Can you work these out from the model? Positions are in its coordinate system, mm. A direction names the side the tool comes from. Give positions to 0.01 mm unless a question says otherwise; leave off trailing zeros. Order: outer loops, then holes, each group sorted by start corner. A loop starts at its lowest first (then second) coordinate and runs counter-clockwise, first axis right, second up. Notation, with made-up numbers: (33.25, 56) - (69.25, 56) arc R5 cw to (69.25, 62) - close; hole circle Ø11 at (2.5, -31). An arc over 180 degrees is marked (long way). Use one line per item in the form item = value. Start each with the question number.
1) Suppose I cut it at A-A, the plane y = 17. Write out the boundary of the cut face in (x, z).
2) Which directions (+Z, -Z, +X, -X, +Y, -Y) give clear straight access to the entire face, cutting with the end or side of a thin tool? Please do faces 1 (the cylindrical face through (-0.22, 5.27, 1.97)), 2 (the flat face through (0, -26.786, 2)), 3 (the flat face through (-1, -14, 4)).
3) For pin 1 (2 mm diameter, centred on x = -14, z = 0.5, fed in from +Y); pin 2 (1.5 mm diameter, centred on x = -5, z = 3, fed in from -Y), each with a flat end and sliding along its axis, tell me the tip position at first contact or that it passes through.
4) Suppose I cut it at C-C, the plane z = 1.7. Write out the boundary of the cut face in (x, y), and give its area (3 significant figures).
5) Please list where these lines run through material, in increasing order: probe 1 along X at (y, z) = (20.5, 3.75); probe 2 along X at (y, z) = (0.5, 0.9); probe 3 along Y at (x, z) = (-24.5, 1.8).
6) Suppose I cut it at D-D, the plane y = 8. Write out the boundary of the cut face in (x, z).
7) We'd pull the mould along Y, two halves only. Please class faces 4 (the cylindrical face through (-35.992, -25.881, 1.972)), 5 (the flat face through (0, -13.786, 2)), 6 (the flat face through (-1, -14, 0)): released by +Y, released by -Y, zero draft, split by the parting line, or undercut.
8) Suppose I cut it at B-B, the plane x = 6.5. Write out the boundary of the cut face in (y, z), and give its area (3 significant figures).
```python
from build123d import *

# Parameters (mm, degrees)
SKETCH_1_R      = 5.2
EXTRUDE_1_DEPTH = 4


with BuildPart() as part:
    # 草图1 → 凸台-拉伸1 (new body)
    with BuildSketch(Plane.XY):
        with BuildLine():
            Line((-18.494622549, 4.742999843), (-23.409453688, -3.769737399))
            ThreePointArc((-23.409453688, -3.769737399), (-35.781809628, -26.257000157), (-10.121090849, -26.785856986))
            Line((-10.121090849, -26.785856986), (-0.291428571, -26.785856986))
            Line((-0.291428571, -26.785856986), (9.538233706, -26.785856986))
            ThreePointArc((9.538233706, -26.785856986), (35.198952485, -26.257000157), (22.826596545, -3.769737399))
            Line((22.826596545, -3.769737399), (17.911765406, 4.742999843))
            Line((17.911765406, 4.742999843), (12.996934268, 13.255737086))
            ThreePointArc((12.996934268, 13.255737086), (-0.291428571, 35.214143014), (-13.579791411, 13.255737086))
            Line((-13.579791411, 13.255737086), (-18.494622549, 4.742999843))
        make_face()
        with Locations((-0.291428571, 20.214143014)):
            Circle(SKETCH_1_R, mode=Mode.SUBTRACT)
        with Locations((22.208571429, -18.757000157)):
            Circle(SKETCH_1_R, mode=Mode.SUBTRACT)
        with Locations((-22.791428571, -18.757000157)):
            Circle(SKETCH_1_R, mode=Mode.SUBTRACT)
        with BuildLine():
            Line((9.268171867, -6.285856986), (4.038698447, 2.771856673))
            ThreePointArc((4.038698447, 2.771856673), (-0.291428571, 5.271856673), (-4.62155559, 2.771856673))
            Line((-4.62155559, 2.771856673), (-9.85102901, -6.285856986))
            ThreePointArc((-9.85102901, -6.285856986), (-9.85102901, -11.285856986), (-5.520901991, -13.785856986))
            Line((-5.520901991, -13.785856986), (4.938044848, -13.785856986))
            ThreePointArc((4.938044848, -13.785856986), (9.268171867, -11.285856986), (9.268171867, -6.285856986))
        make_face(mode=Mode.SUBTRACT)
    extrude(amount=EXTRUDE_1_DEPTH)


solid = part.part
```
Result sheet:
q1.outline = (-14.94, 0) - (-4.38, 0) - (-4.38, 4) - (-14.94, 4) - close; (3.8, 0) - (14.36, 0) - (14.36, 4) - (3.8, 4) - close
q2.face_1 = +Z, -Z
q2.face_2 = +Z, -Z, -Y
q2.face_3 = +Z, +X, -X, +Y, -Y
q3.pin_1 = 28.18
q3.pin_2 = -26.79
q4.outline = (-23.41, -3.77) arc R15 ccw (long way) to (-10.12, -26.79) - (9.54, -26.79) arc R15 ccw (long way) to (22.83, -3.77) - (13, 13.26) arc R15 ccw (long way) to (-13.58, 13.26) - close; hole circle Ø10.4 at (-22.79, -18.76); hole (-9.85, -6.29) arc R5 ccw to (-5.52, -13.79) - (4.94, -13.79) arc R5 ccw to (9.27, -6.29) - (4.04, 2.77) arc R5 ccw to (-4.62, 2.77) - close; hole circle Ø10.4 at (-0.29, 20.21); hole circle Ø10.4 at (22.21, -18.76)
q4.area = 2,500 mm²
q5.probe_1 = -15.29 to -5.48, 4.9 to 14.71
q5.probe_2 = -20.94 to -5.93, 5.35 to 20.36
q5.probe_3 = -33.66 to -23.67, -13.85 to -3.85
q6.outline = (-16.61, 0) - (16.03, 0) - (16.03, 4) - (-16.61, 4) - close
q7.face_4 = split by the parting line
q7.face_5 = undercut
q7.face_6 = zero draft
q8.outline = (-26.79, 0) - (-13.54, 0) - (-13.54, 4) - (-26.79, 4) - close; (-1.49, 0) - (33.59, 0) - (33.59, 4) - (-1.49, 4) - close
q8.area = 193 mm²
